The listing builds one solid part. Answer for the finished solid, in the listing's coordinates (mm). A direction names the side the tool comes from. Round coordinates to 2 decimals unless told otherwise and drop trailing zeros. Loops run counter-clockwise (first coordinate to the right, second up) from the corner with the lowest first, then second, coordinate; pieces in that order, holes last. Notation, with made-up numbers: (31.5, 40) -> (42.5, 40) arc R18 ccw to (42.5, 67) -> close; hole circle Ø4 at (-18.75, 29). An arc over 180 degrees is marked (long way). Answer in a Markdown table with one row per item. Add a question column.
```python
from build123d import *
from build123d.topology import SkipClean

# Parameters (mm, degrees)
SKETCH3_R                = 1.25
BOSS_EXTRUDE2_DEPTH      = 3
BOSS_EXTRUDE3_DEPTH      = 7
BOSS_EXTRUDE3_DEPTH_BACK = 7
CUT_EXTRUDE1_DEPTH       = 67.575853844
BOSS_EXTRUDE4_DEPTH      = 3.5
BOSS_EXTRUDE5_DEPTH      = 4
SKETCH9_R                = 2
BOSS_EXTRUDE6_DEPTH      = 2.5
BOSS_EXTRUDE7_START      = -24
SKETCH10_R               = 1.25
BOSS_EXTRUDE7_DEPTH      = 24
CUT_EXTRUDE2_DEPTH       = 1.5
BOSS_EXTRUDE8_START      = 2.5
SKETCH12_R               = 1.25
BOSS_EXTRUDE8_DEPTH      = 2.5


with BuildPart() as part:
    # Sketch3 → Boss-Extrude2 (new body)
    with BuildSketch(Plane.XY):
        with BuildLine():
            Line((-58.067604658, 9.129873432), (-17.927673113, 9.129873432))
            ThreePointArc((-17.927673113, 9.129873432), (-17.144364104, 9.003989478), (-16.439939924, 8.63901503))
            Line((-16.439939924, 8.63901503), (-9.662890391, 3.620731835))
            ThreePointArc((-9.662890391, 3.620731835), (-8.958466211, 3.255757387), (-8.175157202, 3.129873432))
            Line((-8.175157202, 3.129873432), (8.175157202, 3.129873432))
            ThreePointArc((8.175157202, 3.129873432), (8.958466211, 3.255757387), (9.662890391, 3.620731835))
            Line((9.662890391, 3.620731835), (16.439939924, 8.63901503))
            ThreePointArc((16.439939924, 8.63901503), (17.144364104, 9.003989478), (17.927673113, 9.129873432))
            Line((17.927673113, 9.129873432), (58.024732939, 9.129873432))
            ThreePointArc((58.024732939, 9.129873432), (60.713666824, 8.091230311), (62.006179367, 5.514690714))
            Line((62.006179367, 5.514690714), (62.485680247, 0.553616565))
            ThreePointArc((62.485680247, 0.553616565), (59.4550541, -5.663918261), (53.112535099, -2.904409812))
            ThreePointArc((53.112535099, -2.904409812), (52.191454269, -1.788745789), (50.80658819, -1.370126568))
            Line((50.80658819, -1.370126568), (29.971601132, -1.370126568))
            ThreePointArc((29.971601132, -1.370126568), (29.266449795, -1.471635044), (28.618561527, -1.767917294))
            Line((28.618561527, -1.767917294), (21.476313645, -6.364864122))
            ThreePointArc((21.476313645, -6.364864122), (21.063134423, -6.579260655), (20.617370927, -6.713342154))
            Line((20.617370927, -6.713342154), (0.494096887, -10.770508908))
            ThreePointArc((0.494096887, -10.770508908), (0, -10.819821603), (-0.494096887, -10.770508908))
            Line((-0.494096887, -10.770508908), (-20.617370927, -6.713342154))
            ThreePointArc((-20.617370927, -6.713342154), (-21.063134423, -6.579260655), (-21.476313645, -6.364864122))
            Line((-21.476313645, -6.364864122), (-28.618561527, -1.767917294))
            ThreePointArc((-28.618561527, -1.767917294), (-29.266449795, -1.471635044), (-29.971601132, -1.370126568))
            Line((-29.971601132, -1.370126568), (-50.80658819, -1.370126568))
            ThreePointArc((-50.80658819, -1.370126568), (-52.191454269, -1.788745789), (-53.112535099, -2.904409812))
            ThreePointArc((-53.112535099, -2.904409812), (-58.972993776, -5.814575808), (-62.69520812, -0.433204011))
            Line((-62.69520812, -0.433204011), (-62.044228019, 5.561691263))
            ThreePointArc((-62.044228019, 5.561691263), (-60.739002108, 8.107059295), (-58.067604658, 9.129873432))
        make_face()
        with Locations((0, -6.620126568)):
            Circle(SKETCH3_R, mode=Mode.SUBTRACT)
        with Locations((-57.724428918, -0.9729763)):
            Circle(SKETCH3_R, mode=Mode.SUBTRACT)
        with Locations(Location((57.724428918, -0.9729763, 0), (0, 0, 180))):
            Circle(SKETCH3_R, mode=Mode.SUBTRACT)
        with Locations((-20.303113823, 3.613972241)):
            Circle(SKETCH3_R, mode=Mode.SUBTRACT)
        with Locations((-17.030694447, 1.32049797)):
            Circle(SKETCH3_R, mode=Mode.SUBTRACT)
        with Locations((-13.758275071, -0.9729763)):
            Circle(SKETCH3_R, mode=Mode.SUBTRACT)
        with Locations(Location((13.758275071, -0.9729763, 0), (0, 0, 180))):
            Circle(SKETCH3_R, mode=Mode.SUBTRACT)
        with Locations(Location((17.030694447, 1.32049797, 0), (0, 0, 180))):
            Circle(SKETCH3_R, mode=Mode.SUBTRACT)
        with Locations(Location((20.303113823, 3.613972241, 0), (0, 0, 180))):
            Circle(SKETCH3_R, mode=Mode.SUBTRACT)
    extrude(amount=BOSS_EXTRUDE2_DEPTH)

    # Sketch5 → Boss-Extrude3 (add, two sides: drawn at the far end of the back side and taken through both)
    with BuildSketch(Plane.XY.offset(3).offset(-BOSS_EXTRUDE3_DEPTH_BACK)):
        with BuildLine():
            ThreePointArc((-17.630126475, 7.031701752), (-17.771011311, 7.104696641), (-17.927673113, 7.129873432))
            Line((-17.927673113, 7.129873432), (-58.067604658, 7.129873432))
            Line((-58.067604658, 7.129873432), (-58.067604658, 9.129873432))
            Line((-58.067604658, 9.129873432), (-17.927673113, 9.129873432))
            ThreePointArc((-17.927673113, 9.129873432), (-17.144364104, 9.003989478), (-16.439939924, 8.63901503))
            Line((-16.439939924, 8.63901503), (-9.662890391, 3.620731835))
            ThreePointArc((-9.662890391, 3.620731835), (-8.958466211, 3.255757387), (-8.175157202, 3.129873432))
            Line((-8.175157202, 3.129873432), (8.175157202, 3.129873432))
            ThreePointArc((8.175157202, 3.129873432), (8.958466211, 3.255757387), (9.662890391, 3.620731835))
            Line((9.662890391, 3.620731835), (16.439939924, 8.63901503))
            ThreePointArc((16.439939924, 8.63901503), (17.144364104, 9.003989478), (17.927673113, 9.129873432))
            Line((17.927673113, 9.129873432), (58.024732939, 9.129873432))
            Line((58.024732939, 9.129873432), (58.024732939, 7.129873432))
            Line((58.024732939, 7.129873432), (17.927673113, 7.129873432))
            ThreePointArc((17.927673113, 7.129873432), (17.771011311, 7.104696641), (17.630126475, 7.031701752))
            Line((17.630126475, 7.031701752), (10.853076942, 2.013418557))
            ThreePointArc((10.853076942, 2.013418557), (9.585113418, 1.356464551), (8.175157202, 1.129873432))
            Line((8.175157202, 1.129873432), (-8.175157202, 1.129873432))
            ThreePointArc((-8.175157202, 1.129873432), (-9.585113418, 1.356464551), (-10.853076942, 2.013418557))
            Line((-10.853076942, 2.013418557), (-17.630126475, 7.031701752))
        make_face()
    extrude(amount=BOSS_EXTRUDE3_DEPTH + BOSS_EXTRUDE3_DEPTH_BACK)

    # Sketch6 → Cut-Extrude1 (cut, through all)
    with BuildSketch(Plane(origin=(0, 9.129873432, 0), x_dir=(1, 0, 0), z_dir=(0, 1, 0))):
        with BuildLine():
            Line((-58.067604658, 0), (-41.667544995, 3.748585066))
            ThreePointArc((-41.667544995, 3.748585066), (-40.560490394, 3.936947485), (-39.43929698, 4))
            Line((-39.43929698, 4), (-58.067604658, 4))
            Line((-58.067604658, 4), (-58.067604658, 0))
        make_face()
        with BuildLine():
            Line((-58.067604658, -4.546629265), (-9.076321467, -9.93994917))
            ThreePointArc((-9.076321467, -9.93994917), (-8.530013446, -9.984976007), (-7.982058932, -10))
            Line((-7.982058932, -10), (-58.067604658, -10))
            Line((-58.067604658, -10), (-58.067604658, -4.546629265))
        make_face()
        with BuildLine():
            Line((58.067604658, -10), (58.067604658, -4.546629265))
            Line((58.067604658, -4.546629265), (9.076321467, -9.93994917))
            ThreePointArc((9.076321467, -9.93994917), (8.530013446, -9.984976007), (7.982058932, -10))
            Line((7.982058932, -10), (58.067604658, -10))
        make_face()
        with BuildLine():
            Line((58.067604658, 4), (58.067604658, 0))
            Line((58.067604658, 0), (41.667544995, 3.748585066))
            ThreePointArc((41.667544995, 3.748585066), (40.560490394, 3.936947485), (39.43929698, 4))
            Line((39.43929698, 4), (58.067604658, 4))
        make_face()
    extrude(amount=-CUT_EXTRUDE1_DEPTH, mode=Mode.SUBTRACT)

    # Sketch7 → Boss-Extrude4 (add)
    with BuildSketch(Plane.XY.offset(3)):
        with BuildLine():
            Line((-62.62884704, 0), (-62.044228019, 5.561691263))
            ThreePointArc((-62.044228019, 5.561691263), (-58.292178075, 9.123564304), (-54.164461461, 6.004786676))
            Line((-54.164461461, 6.004786676), (-52.845499921, 0.120665255))
            ThreePointArc((-52.845499921, 0.120665255), (-57.66276491, -5.972596041), (-62.62884704, 0))
        make_face()
        with BuildLine():
            Line((-56.116033059, 5.567330054), (-54.79707152, -0.316791367))
            ThreePointArc((-54.79707152, -0.316791367), (-57.727240857, -3.972974982), (-60.65055107, -0.311304821))
            Line((-60.65055107, -0.311304821), (-60.055607169, 5.348610756))
            ThreePointArc((-60.055607169, 5.348610756), (-58.178470954, 7.126798234), (-56.116033059, 5.567330054))
        make_face(mode=Mode.SUBTRACT)
    boss_extrude4 = extrude(amount=BOSS_EXTRUDE4_DEPTH)

    # Mirror1: Boss-Extrude4 across plane
    with SkipClean():  # the faces are left unmerged after this step: merging them gives an invalid solid
        add(boss_extrude4.mirror(Plane(origin=(0, 0, 0), x_dir=(0, 0, 1), z_dir=(1, 0, 0))))

    # Sketch8 → Boss-Extrude5 (add)
    with SkipClean():  # the faces are left unmerged after this step: merging them gives an invalid solid
        with BuildSketch(Plane(origin=(0, 0, -4), x_dir=(-1, 0, 0), z_dir=(0, 0, -1))):
            with BuildLine():
                Line((-23.819015015, 3.613972241), (-24.838972745, 3.613972241))
                Line((-24.838972745, 3.613972241), (-24.838972745, 7.129873432))
                Line((-24.838972745, 7.129873432), (-20.303113823, 7.129873432))
                ThreePointArc((-20.303113823, 7.129873432), (-22.789231398, 6.100089815), (-23.819015015, 3.613972241))
            make_face()
            with BuildLine():
                Line((24.838972745, 7.129873432), (20.303113823, 7.129873432))
                ThreePointArc((20.303113823, 7.129873432), (22.789231398, 6.100089815), (23.819015015, 3.613972241))
                Line((23.819015015, 3.613972241), (24.838972745, 3.613972241))
                Line((24.838972745, 3.613972241), (24.838972745, 7.129873432))
            make_face()
        extrude(amount=-BOSS_EXTRUDE5_DEPTH)

    # Sketch9 → Boss-Extrude6 (add)
    with SkipClean():  # the faces are left unmerged after this step: merging them gives an invalid solid
        with BuildSketch(Plane.XY.offset(3)):
            with Locations((17.030694447, 1.32049797)):
                Circle(SKETCH9_R)
        boss_extrude6 = extrude(amount=BOSS_EXTRUDE6_DEPTH)

    # Sketch10 → Boss-Extrude7 (add)
    with SkipClean():  # the faces are left unmerged after this step: merging them gives an invalid solid
        with BuildSketch(Plane.XY.offset(5.5).offset(BOSS_EXTRUDE7_START)):
            with Locations((17.030694447, 1.32049797)):
                Circle(SKETCH10_R)
        boss_extrude7 = extrude(amount=BOSS_EXTRUDE7_DEPTH)

    # Sketch11 → Cut-Extrude2 (cut)
    with SkipClean():  # the faces are left unmerged after this step: merging them gives an invalid solid
        with BuildSketch(Plane.XY.offset(5.5)):
            Polygon((17.827404099, 2.700439566), (16.233984796, 2.700439566), (15.437275144, 1.32049797), (16.233984796, -0.059443625), (17.827404099, -0.059443625), (18.62411375, 1.32049797), align=None)
        cut_extrude2 = extrude(amount=-CUT_EXTRUDE2_DEPTH, mode=Mode.SUBTRACT)

    # Sketch12 → Boss-Extrude8 (add)
    with SkipClean():  # the faces are left unmerged after this step: merging them gives an invalid solid
        with BuildSketch(Plane(origin=(0, 0, 0), x_dir=(-1, 0, 0), z_dir=(0, 0, -1)).offset(BOSS_EXTRUDE8_START)):
            Polygon((-15.29864364, 4.32049797), (-18.762745255, 4.32049797), (-20.494796062, 1.32049797), (-18.762745255, -1.67950203), (-15.29864364, -1.67950203), (-13.566592832, 1.32049797), align=None)
            with Locations(Location((-17.030694447, 1.32049797, 0), (0, 0, 180))):
                Circle(SKETCH12_R, mode=Mode.SUBTRACT)
        boss_extrude8 = extrude(amount=-BOSS_EXTRUDE8_DEPTH)

    # Mirror2: Boss-Extrude6, Boss-Extrude7, Cut-Extrude2, Boss-Extrude8 across plane
    with SkipClean():  # the faces are left unmerged after this step: merging them gives an invalid solid
        add(boss_extrude6.mirror(Plane(origin=(0, 0, 0), x_dir=(0, 0, 1), z_dir=(1, 0, 0))))
        add(boss_extrude7.mirror(Plane(origin=(0, 0, 0), x_dir=(0, 0, 1), z_dir=(1, 0, 0))))
        add(cut_extrude2.mirror(Plane(origin=(0, 0, 0), x_dir=(0, 0, 1), z_dir=(1, 0, 0))), mode=Mode.SUBTRACT)
        add(boss_extrude8.mirror(Plane(origin=(0, 0, 0), x_dir=(0, 0, 1), z_dir=(1, 0, 0))))


solid = part.part
```
Item 1: Consider L1, parallel to X at y = -2.5, z = 0.25; L2, parallel to Y at x = -1, z = 3.25; L3, parallel to Z at x = 5.5, y = 1.75. Determine where each line is inside the solid, lowest interval first. Write a range as from..to.
Item 2: For faces 5 (the flat face through (13, 6.09, 2.84)), 6 (the cylindrical face through (21.55, 3.56, 1.48)), 7 (the flat face through (-61, 2, 6.5)), 8 (the flat face through (-40, -1.37, 1)), 9 (the cylindrical face through (9.6, 1.36, 6.45)), determine the directions among +Z, -Z, +X, -X, +Y, -Y from which every point of the face is accessible in a straight line to the end or side of a thin tool.
Item 3: Section A-A, the plane z = -13.5 is taken. Write down the section's boundary in (x, y), and give its area (3 significant figures).
Item 4: Flat-ended cylindrical pins translate along their axes: P1, Ø3, axis at x = 25, y = 3.5, coming from the -Z side; P2, Ø1.8, axis at y = 5, z = -1, coming from the +X side; P3, Ø6.5, axis at x = 39.5, z = 5, coming from the -Y side. Find the tip coordinate at first contact, or state that the pin passes through.
Item 5: The mould has two halves that part along X. Classify faces 1 (the cylindrical face through (58.716, -0.212, 1.479)), 2 (the flat face through (-38, 7.13, -2)), 3 (the flat face through (-24.839, 5, -2)), 4 (the flat face through (24.839, 5, -2)): +X half, -X half, draft (parallel to the pull), parting line (faces both ways), or undercut.
Item 6: Section C-C, the plane y = -9 is taken. Write down the section's boundary in (x, z), and give its area (3 significant figures).
Item 7: Section B-B, the plane x = -48.5 is taken. Write down the section's boundary in (y, z).
Here are the results:
| question | item | result |
|---|---|---|
| 1 | L1 | x = -62.49..-52.9, -27.48..27.48, 52.9..62.49 |
| 1 | L2 | y = 1.13..3.13 |
| 1 | L3 | z = -4..10 |
| 2 | face 5 | +Z, -Z, +Y |
| 2 | face 6 | +Z |
| 2 | face 7 | +Z, -X, +Y, -Y |
| 2 | face 8 | +Z, -Z, -Y |
| 2 | face 9 | +Z, -Y |
| 3 | outline | circle Ø2.5 at (-17.03, 1.32); circle Ø2.5 at (17.03, 1.32) |
| 3 | area | 9.82 mm² |
| 4 | P1 | stops at z = -4 |
| 4 | P2 | stops at x = 24.84 |
| 4 | P3 | stops at y = -1.37 |
| 5 | face 1 | undercut |
| 5 | face 2 | draft |
| 5 | face 3 | -X half |
| 5 | face 4 | +X half |
| 6 | outline | (-9.28, 0) -> (9.28, 0) -> (9.28, 3) -> (-9.28, 3) -> close |
| 6 | area | 55.7 mm² |
| 7 | outline | (-1.37, 0) -> (7.13, 0) -> (7.13, -2.19) -> (9.13, -2.19) -> (9.13, 5.6) -> (7.13, 5.6) -> (7.13, 3) -> (-1.37, 3) -> close |
